Could you check a few things on this drawing? It's one solid part, dimensions in mm from its lowest x, y, z. A direction names the side the tool comes from. Give positions to 0.01 mm unless a question says otherwise; leave off trailing zeros. Order: outer loops, then holes, each group sorted by start corner. A loop starts at its lowest first (then second) coordinate and runs counter-clockwise, first axis right, second up. Notation, with made-up numbers: (29.5, 74) - (72.5, 74) arc R26 cw to (72.5, 96) - close; hole circle Ø6 at (-5.5, 55). An arc over 180 degrees is marked (long way). Put each result on its own line as item: value.
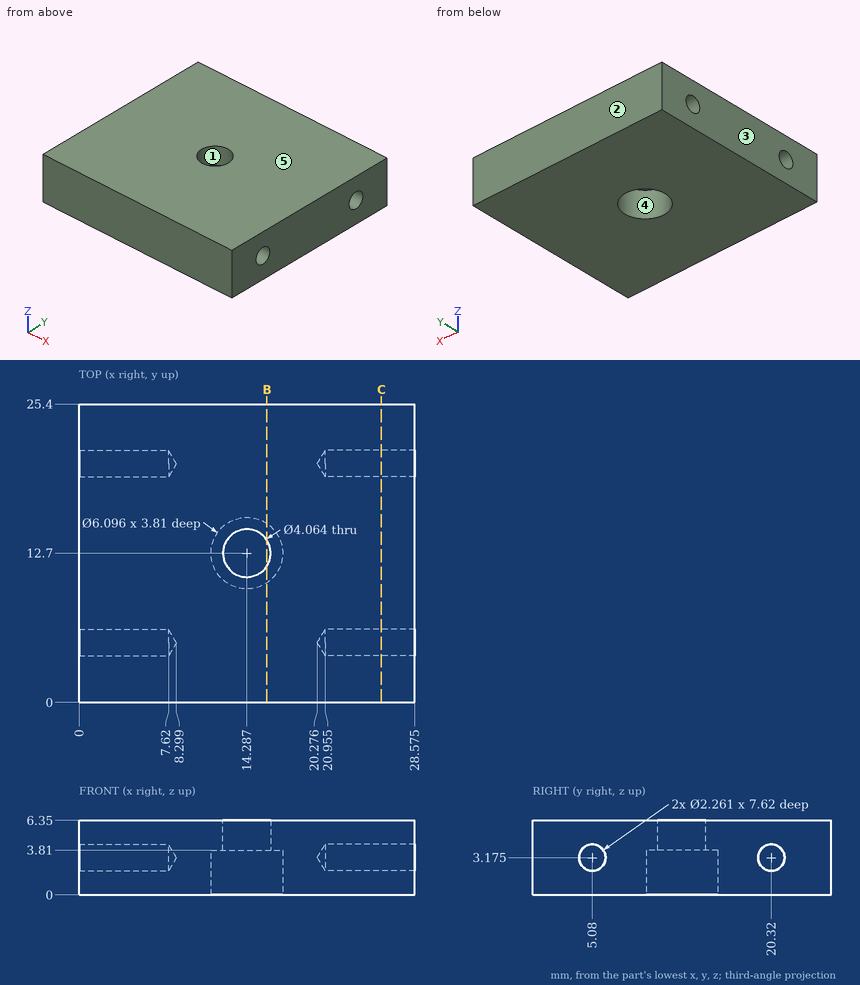
1) I'm going to push flat-ended pins straight in: pin 1 (1 mm diameter, centred on y = 20.5, z = 4.5, fed in from -X); pin 2 (1.8 mm diameter, centred on y = 5.08, z = 3.175, fed in from -X); pin 3 (3 mm diameter, centred on x = 13.5, y = 12, fed in from -Z); pin 4 (1.8 mm diameter, centred on y = 5.08, z = 3.175, fed in from +X). Where does each tip first touch, or does it pass through?
Filled in:
pin 1: stops at x = 0
pin 2: stops at x = 7.76
pin 3: stops at z = 3.81
pin 4: stops at x = 20.82
2) If I drill on line 1 (X direction, y = 13, z = 1) (1 decimal); line 2 (Y direction, x = 25.25, z = 2.5) (1 decimal); line 3 (X direction, y = 13.5, z = 2.25) (1 decimal), over which ranges is the centre line in solid material (lowest first)? Write a range as [from, to].
Filled in:
line 1: x = [0, 11.3], [17.3, 28.6]
line 2: y = [0, 4.2], [6, 19.4], [21.2, 25.4]
line 3: x = [0, 11.3], [17.2, 28.6]
3) Suppose I cut it at C-C, the plane x = 25.75. State how many separate pieces and enclosed holes the cut face has, and give its area (3 significant figures).
Filled in:
separate pieces: 1
enclosed holes: 2
area: 153 mm^2
4) Suppose I cut it at B-B, the plane x = 16. List the corners of the cut face in (y, z) for me.
Filled in:
outline: (0, 0) - (10.18, 0) - (10.18, 3.81) - (11.61, 3.81) - (11.61, 6.35) - (0, 6.35) - close; (13.79, 3.81) - (15.22, 3.81) - (15.22, 0) - (25.4, 0) - (25.4, 6.35) - (13.79, 6.35) - close
5) Which directions (+Z, -Z, +X, -X, +Y, -Y) give clear straight access to the entire face, cutting with the end or side of a thin tool? Please do the marked faces 4 and 5.
Filled in:
face 4: -Z
face 5: +Z, +X, -X, +Y, -Y
6) We'd pull the mould along X, two halves only. Please class the marked faces 1, 2 and 3: pulls with the +X half, pulls with the -X half, needs draft (parallel to the pull), parting line crosses it, or undercut.
Filled in:
face 1: undercut
face 2: needs draft
face 3: pulls with the -X half
